Model file for the job. Use its own axes, mm. A direction names the side the tool comes from. Give positions to 0.01 mm unless a question says otherwise; leave off trailing zeros. Write each loop counter-clockwise with the first axis right and the second up, starting at its lowest first coordinate (ties: lowest second). Pieces come first, ordered by that corner, then holes. Notation, with made-up numbers: M -18.75,49 L 7.25,49 A16 cw 7.25,77 Z; hole C 88.25,1.5 d3. An arc over 180 degrees is marked long. Answer as a JSON object with one key per item and string values. Group by question number.
```python
from build123d import *

# Parameters (mm, degrees)
ESBO_O1_W                = 420
ESBO_O1_H                = 420
ESBO_O1_W_2              = 410
ESBO_O1_H_2              = 410
RESSALTO_EXTRUS_O1_DEPTH = 432
ESBO_O4_R                = 2.5
RESSALTO_EXTRUS_O4_DEPTH = 183.55
ESBO_O4_4_R              = 2.5
RESSALTO_EXTRUS_O5_DEPTH = 188.55
ESBO_O5_R                = 2.5
RESSALTO_EXTRUS_O6_DEPTH = 183.45
ESBO_O6_R                = 15
RESSALTO_EXTRUS_O7_DEPTH = 183.45


with BuildPart() as part:
    # Esboço1 → Ressalto-extrusão1 (new body)
    with BuildSketch(Plane.XY):
        Rectangle(ESBO_O1_W, ESBO_O1_H)
        Rectangle(ESBO_O1_W_2, ESBO_O1_H_2, mode=Mode.SUBTRACT)
    extrude(amount=RESSALTO_EXTRUS_O1_DEPTH)

    # Esboço4 → Ressalto-extrusão4 (add)
    with BuildSketch(Plane.ZY.offset(210)):
        with Locations((400.68, 72.17)):
            Circle(ESBO_O4_R)
    extrude(amount=-RESSALTO_EXTRUS_O4_DEPTH)

    # Esboço4<4> → Ressalto-extrusão5 (add)
    with BuildSketch(Plane.ZY.offset(210)):
        with Locations((347.87, 58.16)):
            Circle(ESBO_O4_4_R)
    extrude(amount=-RESSALTO_EXTRUS_O5_DEPTH)

    # Esboço5 → Ressalto-extrusão6 (add)
    with BuildSketch(Plane(origin=(210, 0, 0), x_dir=(0, 0, -1), z_dir=(1, 0, 0))):
        with Locations((-353.49, 138.09)):
            Circle(ESBO_O5_R)
        with Locations((-427.35, 75.92)):
            Circle(ESBO_O5_R)
    extrude(amount=-RESSALTO_EXTRUS_O6_DEPTH)

    # Esboço6 → Ressalto-extrusão7 (add)
    with BuildSketch(Plane.ZY.offset(210)):
        with Locations((150.03, -10.05)):
            Circle(ESBO_O6_R)
    extrude(amount=-RESSALTO_EXTRUS_O7_DEPTH)


solid = part.part
```
Q1. Slice it at C-C, the plane z = 237. Write the cut outline in (x, y).
Q2. 3-axis set-ups, long thin cutter, end or side, ignore diameter. For faces 1 (the flat face through (-3, -205, 213)), 2 (the cylindrical face through (-117.024, -5.544, 164.337)), 3 (the flat face through (-210, 3, 213)): which of +Z, -Z, +X, -X, +Y, -Y reach the whole face in a straight line?
Q3. Two-plate mould, pull along X, no slides. Class faces 4 (the flat face through (-3, 210, 213)), 5 (the flat face through (210, 3, 219)), 6 (the flat face through (-205, -3, 213)): +X half, -X half, draft (parallel to the pull), parting line (faces both ways), or undercut.
Q4. Slice it at D-D, the plane x = -54.5. Write the cut outline in (y, z).
Q5. Wall check: L1, parallel to Y at x = -131, z = 148; L2, parallel to Y at x = 133.5, z = 159. Give the ranges that are in metal, low to high.
Q6. Slice it at A-A, the plane y = -10.05. Write the cut outline in (x, z), then the cut area to 3 significant figures.
Q7. Slice it at B-B, the plane x = 165. Write the cut outline in (y, z), then the cut area to 3 significant figures.
Solved:
{
 "1": {"outline": "M -210,-210 L 210,-210 L 210,210 L -210,210 Z; hole M -205,-205 L 205,-205 L 205,205 L -205,205 Z"},
 "2": {"face 1": "+Z, -Z", "face 2": "none", "face 3": "+Z, -Z, -X, +Y, -Y"},
 "3": {"face 4": "draft", "face 5": "+X half", "face 6": "undercut"},
 "4": {"outline": "M -210,0 L -205,0 L -205,432 L -210,432 Z; C -10.05,150.03 d30; C 58.16,347.87 d5; C 72.17,400.68 d5; M 205,0 L 210,0 L 210,432 L 205,432 Z"},
 "5": {"L1": "y = -210 to -205, -24.91 to 4.81, 205 to 210", "L2": "y = -210 to -205, 205 to 210"},
 "6": {"outline": "M -210,0 L -205,0 L -205,135.03 L -26.55,135.03 L -26.55,165.03 L -205,165.03 L -205,432 L -210,432 Z; M 205,0 L 210,0 L 210,432 L 205,432 Z", "area": "9,670 mm²"},
 "7": {"outline": "M -210,0 L -205,0 L -205,432 L -210,432 Z; C 75.92,427.35 d5; C 138.09,353.49 d5; M 205,0 L 210,0 L 210,432 L 205,432 Z", "area": "4,360 mm²"}
}
